For this review, use the dimensioned drawing (mm, ordinates from the lowest corner) and the shaded views. A direction names the side the tool comes from. Coordinates: 2 decimals unless noted, no trailing zeros. Loops run counter-clockwise (first coordinate to the right, second up) from the corner with the lowest first, then second, coordinate; pieces in that order, holes last. Notation, with made-up numbers: M 23,45.5 L 80,45.5 A18 ccw 80,74.5 Z; hole C 52.25,-22.75 d9. An arc over 180 degrees is marked long. Use CSV: the item, a comma, the result in double quotes. Start each with the question number.
1. Add section A-A, the plane z = 20. Write out the cut boundary in (x, y).
2. Add section C-C, the plane x = 10.5. Write out the cut boundary in (y, z), then the cut area to 3 significant figures.
3. Tool access review of the marked faces 1, 2 and 3: name each direction out of +Z, -Z, +X, -X, +Y, -Y from which nothing blocks a thin tool from reaching the whole face with its end or side.
4. Clearance check with flat-ended pins moving along their axes: P1, Ø1, axis at x = 5.5, z = 21, coming from the -Y side; P2, Ø6, axis at x = 10.5, y = 25.5, coming from the -Z side; P3, Ø8, axis at x = 3.5, z = 14.5, coming from the +Y side; P4, Ø1.8, axis at y = 20, z = 20, coming from the +X side. State where each tip first meets the part, or that it passes through.
5. For L1, parallel to Z at x = 12.1, y = 20; L2, parallel to Y at x = 10.25, z = 21; L3, parallel to X at y = 20, z = 9, list the stretches that pass through material, from the lowest coordinate up.
6. Add section D-D, the plane y = 36.5. Write out the cut boundary in (x, z), then the cut area to 3 significant figures.
7. Draft analysis for pull direction Y (two halves, no side actions). For the marked faces 4, 5 and 6, state which applies: +Y half, -Y half, draft (parallel to the pull), parting line (faces both ways), or undercut.
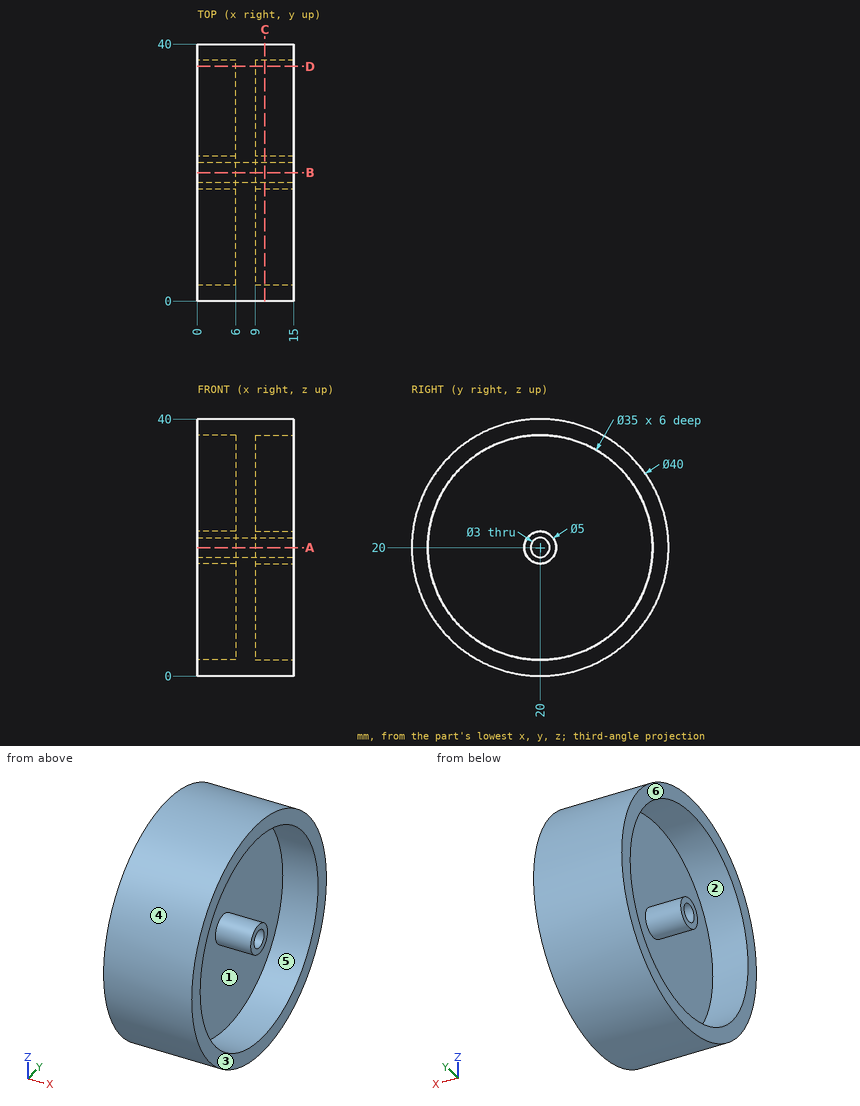
Computed:
1,outline,"M 0,0 L 15,0 L 15,2.5 L 9,2.5 L 9,17.5 L 15,17.5 L 15,18.5 L 0,18.5 L 0,17.5 L 6,17.5 L 6,2.5 L 0,2.5 Z; M 0,21.5 L 15,21.5 L 15,22.5 L 9,22.5 L 9,37.5 L 15,37.5 L 15,40 L 0,40 L 0,37.5 L 6,37.5 L 6,22.5 L 0,22.5 Z"
2,outline,"C 20,20 d40; C 20,20 d5; hole C 20,20 d35; hole C 20,20 d3"
2,area,"307 mm^2"
3,face 1,"+X"
3,face 2,"-X"
3,face 3,"+Z, -Z, +X, +Y, -Y"
4,P1,"stops at y = 0.01"
4,P2,"stops at z = 0.16"
4,P3,"stops at y = 39.94"
4,P4,"passes through"
5,L1,"z = 0 to 2.5, 17.5 to 18.5, 21.5 to 22.5, 37.5 to 40"
5,L2,"y = 0.03 to 2.53, 17.71 to 18.88, 21.12 to 22.29, 37.47 to 39.97"
5,L3,"x = 6 to 9"
6,outline,"M 0,8.7 L 15,8.7 L 15,14.17 L 9,14.17 L 9,25.83 L 15,25.83 L 15,31.3 L 0,31.3 L 0,25.83 L 6,25.83 L 6,14.17 L 0,14.17 Z"
6,area,"199 mm^2"
7,face 4,"parting line"
7,face 5,"undercut"
7,face 6,"draft"
